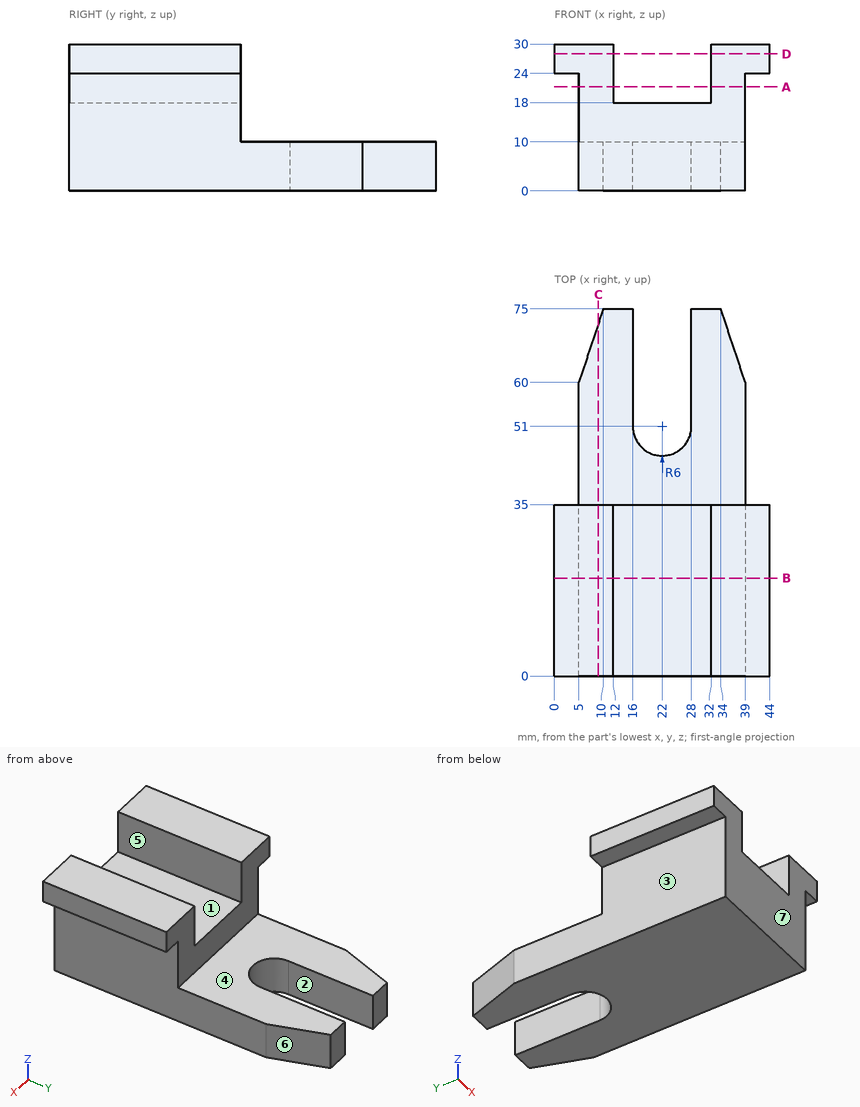
Design review of the part shown in the three views and the two pictorial views. Dimensions are in mm from the part's minimum x, y and z. A direction names the side the tool comes from. Round coordinates to 2 decimals unless told otherwise and drop trailing zeros. Loops run counter-clockwise (first coordinate to the right, second up) from the corner with the lowest first, then second, coordinate; pieces in that order, holes last. Notation, with made-up numbers: (26.5, -29) - (57.5, -29) arc R17 ccw to (57.5, -6) - close; hole circle Ø2 at (15.5, 41.5). An arc over 180 degrees is marked (long way). Use one line per item in the form item = value.
1) Tool access review of the marked faces 1, 2, 3 and 4: name each direction out of +Z, -Z, +X, -X, +Y, -Y from which nothing blocks a thin tool from reaching the whole face with its end or side.
Solutions:
face_1 = +Z, +Y, -Y
face_2 = +Z, -Z, +Y
face_3 = -Z, -X, +Y, -Y
face_4 = +Z, +X, -X, +Y
2) We need section D-D on z = 28. Write out the cut boundary in (x, y), then the cut area to 3 significant figures.
Solutions:
outline = (0, 0) - (12, 0) - (12, 35) - (0, 35) - close; (32, 0) - (44, 0) - (44, 35) - (32, 35) - close
area = 840 mm2
3) We need section C-C on x = 9. Write out the cut boundary in (y, z), then the cut area to 3 significant figures.
Solutions:
outline = (0, 0) - (72, 0) - (72, 10) - (35, 10) - (35, 30) - (0, 30) - close
area = 1,420 mm2
4) We need section A-A on z = 21.25. Write out the cut boundary in (x, y), then the cut area to 3 significant figures.
Solutions:
outline = (5, 0) - (12, 0) - (12, 35) - (5, 35) - close; (32, 0) - (39, 0) - (39, 35) - (32, 35) - close
area = 490 mm2
5) Wall thickness on probe 1 along X at (y, z) = (51, 9.5); probe 2 along X at (y, z) = (12, 27.25); probe 3 along X at (y, z) = (30.5, 2.5): over which ranges is each line inside the solid? List them lowest first.
Solutions:
probe_1 = 5 to 16, 28 to 39
probe_2 = 0 to 12, 32 to 44
probe_3 = 5 to 39
6) We need section B-B on y = 20. Write out the cut boundary in (x, z), then the cut area to 3 significant figures.
Solutions:
outline = (0, 24) - (5, 24) - (5, 0) - (39, 0) - (39, 24) - (44, 24) - (44, 30) - (32, 30) - (32, 18) - (12, 18) - (12, 30) - (0, 30) - close
area = 840 mm2
7) Clearance check with flat-ended pins moving along their axes: P1, Ø4, axis at y = 11.5, z = 13.5, coming from the -X side; P2, Ø6, axis at x = 12, z = 21, coming from the +Y side; P3, Ø10, axis at x = 13.5, y = 45.5, coming from the +Z side. State where each tip first meets the part, or that it passes through.
Solutions:
P1 = 5
P2 = 35
P3 = 10
8) Mouldability with a two-part tool opening along X and no side actions: class the marked faces 5, 6 and 7 as pulls with the +X half, pulls with the -X half, needs draft (parallel to the pull), parting line crosses it, or undercut.
Solutions:
face_5 = undercut
face_6 = pulls with the +X half
face_7 = needs draft
